Verification items for this drawing (mm, ordinates from the low corner). A direction names the side the tool comes from. Round coordinates to 2 decimals unless told otherwise and drop trailing zeros. Order: outer loops, then holes, each group sorted by start corner. A loop starts at its lowest first (then second) coordinate and runs counter-clockwise, first axis right, second up. Notation, with made-up numbers: (12, 50.25) -> (24, 50.25) arc R27 cw to (24, 81.25) -> close; hole circle Ø4 at (-25.5, 47.25). An arc over 180 degrees is marked (long way). Use a Markdown table: item, result. Add a question column.
Item 1: Set-up check for the marked faces 5, 6, 7 and 8: record each of +Z, -Z, +X, -X, +Y, -Y from which the full face is reachable in a straight line by a thin tool's end or side.
Item 2: Mould release check, pull along Y, two halves, no side actions. Record for the marked faces 1, 2, 3 and 4: pulls with the +Y half, pulls with the -Y half, needs draft (parallel to the pull), parting line crosses it, or undercut.
Item 3: Sectioned sample at A-A, the plane x = 5.25. Record the cut outline in (y, z).
Item 4: Sectioned sample at C-C, the plane z = 4.25. Record the cut outline in (x, y).
Item 5: Material ranges on probe 1 along X at (y, z) = (10.75, 6.5); probe 2 along Y at (x, z) = (8.5, 7.75); probe 3 along X at (y, z) = (12.5, 2.25), recorded low to high. Write a range as [from, to].
Item 6: Gauge pin test, flat ends, axial feed: pin 1 Ø0.9 at (y, z) = (1.5, 1.5) entering from +X; pin 2 Ø2 at (x, y) = (11, 10) entering from -Z; pin 3 Ø3.5 at (x, y) = (9.5, 13) entering from -Z. Record the tip position at first contact, or that the pin passes through.
Item 7: Sectioned sample at B-B, the plane y = 5.75. Record the cut outline in (x, z), and give its area (3 significant figures).
Item 8: Sectioned sample at D-D, the plane x = 10.5. Record the cut outline in (y, z).
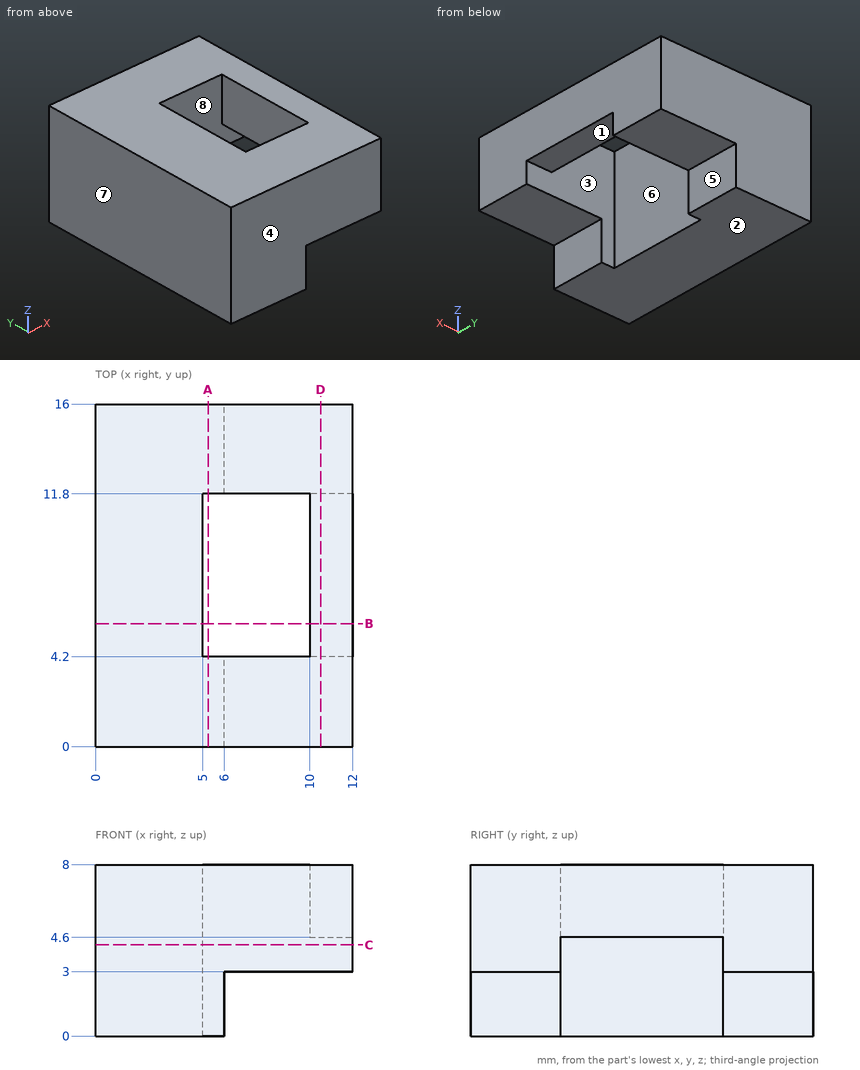
Found:
| question | item | result |
|---|---|---|
| 1 | face 5 | -Z, +X, +Y, -Y |
| 1 | face 6 | +Z, -Z |
| 1 | face 7 | +Z, -Z, -X, +Y, -Y |
| 1 | face 8 | -Z |
| 2 | face 1 | undercut |
| 2 | face 2 | needs draft |
| 2 | face 3 | undercut |
| 2 | face 4 | pulls with the -Y half |
| 3 | outline | (0, 0) -> (4.2, 0) -> (4.2, 8) -> (0, 8) -> close; (11.8, 0) -> (16, 0) -> (16, 8) -> (11.8, 8) -> close |
| 4 | outline | (0, 0) -> (12, 0) -> (12, 4.2) -> (5, 4.2) -> (5, 11.8) -> (12, 11.8) -> (12, 16) -> (0, 16) -> close |
| 5 | probe 1 | x = [0, 5], [10, 12] |
| 5 | probe 2 | y = [0, 4.2], [11.8, 16] |
| 5 | probe 3 | x = [0, 6] |
| 6 | pin 1 | stops at x = 6 |
| 6 | pin 2 | stops at z = 4.6 |
| 6 | pin 3 | stops at z = 3 |
| 7 | outline | (0, 0) -> (5, 0) -> (5, 8) -> (0, 8) -> close; (10, 4.6) -> (12, 4.6) -> (12, 8) -> (10, 8) -> close |
| 7 | area | 46.8 mm2 |
| 8 | outline | (0, 3) -> (4.2, 3) -> (4.2, 4.6) -> (11.8, 4.6) -> (11.8, 3) -> (16, 3) -> (16, 8) -> (0, 8) -> close |
